Work out the finished part from the listing and answer in its coordinate system (mm). A direction names the side the tool comes from. Give positions to 0.01 mm unless a question says otherwise; leave off trailing zeros. Loops run counter-clockwise (first coordinate to the right, second up) from the corner with the lowest first, then second, coordinate; pieces in that order, holes last. Notation, with made-up numbers: (48, 5.5) - (64, 5.5) arc R20 ccw to (64, 41.5) - close; hole circle Ø6 at (8.5, 31). An arc over 180 degrees is marked (long way). One line per question, with ' | ' between items.
from build123d import *

# Parameters (mm, degrees)
F3_R             = 37.5
F4_DEPTH         = 2
F8_R             = 4
F9_DEPTH         = 5
F7_R             = 2.5
F10_DEPTH        = 5
F10_TAPER        = 2
F14_COPIES_COUNT = 2
F16_COPIES_COUNT = 2


# Not quite as in the source:
# - a pattern or mirror of a feature is missing from the dataset's text; its kind, count and spacing are read off the source's solid


with BuildPart() as f2:
    # F1 (on Front) → F2 (revolve)
    with BuildSketch(Plane.XZ):
        with BuildLine():
            Line((-16, 0), (-21.33, 0))
            ThreePointArc((-21.33, 0), (-18.665, -2.665), (-16, 0))
        make_face()
    revolve(axis=Axis((0, 0, 18.396249041), (0, 0, 1)))

    # F3 (on face) → F4 (join)
    with BuildSketch(Plane.XY):
        Circle(F3_R)
    extrude(amount=F4_DEPTH)

    # F5 (on Right) → F6 (revolve)
    with BuildSketch(Plane.YZ):
        Polygon((-36.8366060944, -9.6), (-35.1438670796, 0), (-37.5, 0), (-39.1927390148, -9.6), align=None)
    revolve(axis=Axis((0, 0, 18.396249041), (0, 0, 1)))

    # F8 (on face) → F9 (join)
    with BuildSketch(Plane.XY.offset(2)):
        with Locations((0, -30.5)):
            Circle(F8_R)
        with Locations((26.4137748154, 15.25)):
            Circle(F8_R)
        with Locations((-26.4137748154, 15.25)):
            Circle(F8_R)
    extrude(amount=F9_DEPTH)

    # F7 (on face) → F10 (cut)
    with BuildSketch(Plane(origin=(0, 0, 0), x_dir=(1, 0, 0), z_dir=(0, 0, -1))):
        with Locations((0, 30.5)):
            Circle(F7_R)
        with Locations((-26.4137748154, -15.25)):
            Circle(F7_R)
        with Locations((26.4137748154, -15.25)):
            Circle(F7_R)
    extrude(amount=-F10_DEPTH, taper=F10_TAPER, mode=Mode.SUBTRACT)

    # F13 (on offset) → F14 (join, up to the next surface of F2)
    with BuildSketch(Plane.YZ.offset(33)):
        with BuildLine():
            Line((2.5, 0), (-2.5, 0))
            ThreePointArc((-2.5, 0), (0, -2.5), (2.5, 0))
        make_face()
    f14 = extrude(until=Until.NEXT)

    # F14_copies: F14 ×2 about axis
    f14_copies_axis = Axis((0, 0, 0), (0, 0, 1))
    for i in range(1, F14_COPIES_COUNT):
        add(f14.rotate(f14_copies_axis, i * 360 / F14_COPIES_COUNT))

    # F15 (on offset) → F16 (join, up to the next surface of F2)
    with BuildSketch(Plane.YZ.offset(23)):
        with BuildLine():
            Line((1, 0), (-1, 0))
            ThreePointArc((-1, 0), (0, -1), (1, 0))
        make_face()
    f16 = extrude(until=Until.NEXT, dir=(-1, 0, 0))

    # F16_copies: F16 ×2 about axis
    f16_copies_axis = Axis((0, 0, 0), (0, 0, 1))
    for i in range(1, F16_COPIES_COUNT):
        add(f16.rotate(f16_copies_axis, i * 360 / F16_COPIES_COUNT))

    # F16_face (on face) → F17 section 0
    with BuildSketch(Plane(origin=(23, 0, -0.4244131816), x_dir=(0, 1, 0), z_dir=(1, 0, 0))):
        with BuildLine():
            Line((1, 0.4244131816), (-1, 0.4244131816))
            ThreePointArc((-1, 0.4244131816), (0, -0.5755868184), (1, 0.4244131816))
        make_face()
    # F14_face (on face) → F17 section 1
    with BuildSketch(Plane(origin=(33, 0, -1.0610329539), x_dir=(0, 1, 0), z_dir=(-1, 0, 0))):
        with BuildLine():
            Line((-2.5, -1.0610329539), (2.5, -1.0610329539))
            ThreePointArc((2.5, -1.0610329539), (0, 1.4389670461), (-2.5, -1.0610329539))
        make_face()
    f17 = loft()

    # F17_copies: F17 across plane
    add(f17.mirror(Plane(origin=(0, 0, 0), x_dir=(0, 0, -1), z_dir=(-1, 0, 0))))


solid = f2.part
1. Consider L1, parallel to Z at x = 11.5, y = -7; L2, parallel to X at y = 23, z = -7.25; L3, parallel to X at y = 19, z = -1. Determine where each line is inside the solid, lowest interval first.
Evaluation:
L1: 0 to 2 | L2: -31.22 to -28.24, 28.24 to 31.22 | L3: -32.53 to -29.77, -9.26 to 9.26, 29.77 to 32.53
2. Find section B-B on z = 6. Write down the section's boundary in (x, y), then the cut area to 3 significant figures.
Evaluation:
outline: circle Ø8 at (-26.41, 15.25); circle Ø8 at (0, -30.5); circle Ø8 at (26.41, 15.25) | area: 151 mm2
3. Find section A-A on x = 0. Write down the section's boundary in (y, z) (3 decimals).
Evaluation:
outline: (-39.193, -9.6) - (-36.837, -9.6) - (-35.144, 0) - (-33, 0) - (-32.825, 5) - (-28.175, 5) - (-28, 0) - (-21.33, 0) arc R2.665 ccw to (-16, 0) - (16, 0) arc R2.665 ccw to (21.33, 0) - (35.144, 0) - (36.837, -9.6) - (39.193, -9.6) - (37.5, 0) - (37.5, 2) - (-26.5, 2) - (-26.5, 7) - (-34.5, 7) - (-34.5, 2) - (-37.5, 2) - (-37.5, 0) - close
4. Which of the six approach directions +Z, -Z, +X, -X, +Y, -Y give full straight-line access (tool end or side, diameter ignored) to faces 4 (the flat face through (0, -31, 5)), 5 (the flat face through (0, -30, 7)), 6 (the cylindrical face through (28.6, 18.6, 4.5))?
Evaluation:
face 4: -Z | face 5: +Z, +X, -X, +Y, -Y | face 6: +Z
5. Flat-ended cylindrical pins translate along their axes: pin 1 (8 mm diameter, centred on y = -22, z = -1, fed in from -X); pin 2 (17 mm diameter, centred on x = 6.5, y = 19.5, fed in from -Z) (3 decimals); pin 3 (1 mm diameter, centred on x = -23.5, y = -13.5, fed in from -Z). Find the tip coordinate at first contact, or state that the pin passes through.
Evaluation:
pin 1: x = -33.24 | pin 2: z = -2.665 | pin 3: z = 0
6. Find section D-D on z = -4.25. Write down the section's boundary in (x, y), then the cut area to 3 significant figures.
Evaluation:
outline: circle Ø76.5 at (0, 0); hole circle Ø71.79 at (0, 0) | area: 549 mm2
7. Find section C-C on y = 0. Write down the section's boundary in (x, z) (3 decimals), then the cut area to 3 significant figures.
Evaluation:
outline: (-39.193, -9.6) - (-36.837, -9.6) - (-35.585, -2.5) - (-33, -2.5) - (-23, -1) - (-21.135, -1) arc R2.665 ccw to (-16, 0) - (16, 0) arc R2.665 ccw to (21.135, -1) - (23, -1) - (33, -2.5) - (35.585, -2.5) - (36.837, -9.6) - (39.193, -9.6) - (37.5, 0) - (37.5, 2) - (-37.5, 2) - (-37.5, 0) - close | area: 268 mm2
8. Determine the mould class of faces 1 (the flat face through (-26, 15, 7)), 2 (the cylindrical face through (-0.521, -26.534, 4.465)), 3 (the flat face through (0, 0, 0)) for opening direction X: +X half, -X half, draft (parallel to the pull), parting line (faces both ways), or undercut.
Evaluation:
face 1: draft | face 2: parting line | face 3: undercut
